```python
from build123d import *

# Parameters (mm, degrees)
F0_W     = 91.44
F0_H     = 76.2
F1_DEPTH = 10.16
F3_D     = 4.445
F5_D     = 6.731
F7_DEPTH = 6.35


with BuildPart() as f1:
    # F0 (on Top) → F1 (new body)
    with BuildSketch(Plane.XY):
        Rectangle(F0_W, F0_H)
    extrude(amount=F1_DEPTH)

    # F3 (through all)
    with Locations(Plane.XY.offset(10.16)):
        with Locations((-25.4, 17.78), (25.4, 17.78)):
            Hole(F3_D / 2)

    # F5 (through all)
    with Locations(Plane.XY.offset(10.16)):
        with Locations((-38.1, 28.575), (38.1, 28.575), (-38.1, -28.575), (38.1, -28.575)):
            Hole(F5_D / 2)

    # F6 (on face) → F7 (cut)
    with BuildSketch(Plane.XY):
        Polygon((38.1, 35.503203), (32.1, 32.039102), (32.1, 25.110898), (38.1, 21.646797), (44.1, 25.110898), (44.1, 32.039102), align=None)
        Polygon((-44.1, 25.110898), (-38.1, 21.646797), (-32.1, 25.110898), (-32.1, 32.039102), (-38.1, 35.503203), (-44.1, 32.039102), align=None)
        Polygon((44.1, -25.110898), (38.1, -21.646797), (32.1, -25.110898), (32.1, -32.039102), (38.1, -35.503203), (44.1, -32.039102), align=None)
        Polygon((-32.1, -25.110898), (-38.1, -21.646797), (-44.1, -25.110898), (-44.1, -32.039102), (-38.1, -35.503203), (-32.1, -32.039102), align=None)
    extrude(amount=F7_DEPTH, mode=Mode.SUBTRACT)


solid = f1.part
```
Geometry check sheet. Reference: the model listing, model coordinates, mm. A direction names the side the tool comes from. Give positions to 0.01 mm unless a question says otherwise; leave off trailing zeros. Order: outer loops, then holes, each group sorted by start corner. A loop starts at its lowest first (then second) coordinate and runs counter-clockwise, first axis right, second up.
1. Access from +Z, -Z, +X, -X, +Y, -Y to the whole of each face (thin tool, end or side, straight path). Record for faces 1 (the face through (-26.595, 19.654, 5.009)), 2 (the face through (-41.058, -23.355, 3.131)).
2. Section check A-A, the plane x = 25.4. Enter the section's corners in (y, z), and give its area (3 significant figures).
3. Gauge pin test, flat ends, axial feed: pin 1 Ø3.5 at (x, y) = (39.5, 26) entering from -Z; pin 2 Ø2.5 at (x, y) = (-25.4, 17.78) entering from +Z; pin 3 Ø1.5 at (x, y) = (3, -16) entering from -Z. Record the tip position at first contact, or that the pin passes through.
4. Release check for a two-part mould opening along X. For faces 3 (the face through (-37, 32, 6.35)), 4 (the face through (-1, 1, 10.16)) record: pulls with the +X half, pulls with the -X half, needs draft (parallel to the pull), parting line crosses it, or undercut.
5. Section check C-C, the plane y = 17.78. Enter the section's corners in (x, z).
6. Section check D-D, the plane y = -27. Enter the section's corners in (x, z).
7. Thickness scan on L1, parallel to X at y = 28.5, z = 1.5; L2, parallel to Y at x = -38.1, z = 7.2; L3, parallel to X at y = 30, z = 7.25. Record the ranges inside material, lowest first.
8. Section check B-B, the plane z = 1.5. Give the number of separate pieces and of enclosed holes in the cut face, and give its area (3 significant figures).
Values follow:
1. face 1: +Z, -Z
1. face 2: -Z
2. outline: (-38.1, 0) - (15.56, 0) - (15.56, 10.16) - (-38.1, 10.16) - close; (20, 0) - (38.1, 0) - (38.1, 10.16) - (20, 10.16) - close
2. area: 729 mm2
3. pin 1: stops at z = 6.35
3. pin 2: passes through
3. pin 3: stops at z = 0
4. face 3: undercut
4. face 4: needs draft
5. outline: (-45.72, 0) - (-27.62, 0) - (-27.62, 10.16) - (-45.72, 10.16) - close; (-23.18, 0) - (23.18, 0) - (23.18, 10.16) - (-23.18, 10.16) - close; (27.62, 0) - (45.72, 0) - (45.72, 10.16) - (27.62, 10.16) - close
6. outline: (-45.72, 0) - (-44.1, 0) - (-44.1, 6.35) - (-41.07, 6.35) - (-41.07, 10.16) - (-45.72, 10.16) - close; (-35.13, 6.35) - (-32.1, 6.35) - (-32.1, 0) - (32.1, 0) - (32.1, 6.35) - (35.13, 6.35) - (35.13, 10.16) - (-35.13, 10.16) - close; (41.07, 6.35) - (44.1, 6.35) - (44.1, 0) - (45.72, 0) - (45.72, 10.16) - (41.07, 10.16) - close
7. L1: x = -45.72 to -44.1, -32.1 to 32.1, 44.1 to 45.72
7. L2: y = -38.1 to -31.94, -25.21 to 25.21, 31.94 to 38.1
7. L3: x = -45.72 to -41.15, -35.05 to 35.05, 41.15 to 45.72
8. separate pieces: 1
8. enclosed holes: 6
8. area: 6,440 mm2
